from build123d import *

# Parameters (mm, degrees)
SKETCH_1_W               = 250
SKETCH_1_H               = 250
EXTRUDE_1_DEPTH          = 2
SKETCH_2_W               = 250
SKETCH_2_H               = 125
CUT_EXTRUDE_1_DEPTH      = 2
SKETCH_6_W               = 10
SKETCH_6_H               = 10
EXTRUDE_3_DEPTH          = 10
CUT_EXTRUDE_2_DEPTH      = 125
CUT_EXTRUDE_3_DEPTH      = 178.059312096
CUT_EXTRUDE_3_DEPTH_BACK = 178.059312096


with BuildPart() as part:
    # 草图1 → 凸台-拉伸1 (new body)
    with BuildSketch(Plane(origin=(0, 0, 0), x_dir=(1, 0, 0), z_dir=(0, 1, 0))):
        Rectangle(SKETCH_1_W, SKETCH_1_H)
    extrude(amount=EXTRUDE_1_DEPTH)

    # 草图2 → 切除-拉伸1 (cut)
    with BuildSketch(Plane(origin=(0, 2, 0), x_dir=(1, 0, 0), z_dir=(0, 1, 0))):
        with Locations((0, -62.5)):
            Rectangle(SKETCH_2_W, SKETCH_2_H)
    extrude(amount=-CUT_EXTRUDE_1_DEPTH, mode=Mode.SUBTRACT)

    # 草图6 → 凸台-拉伸3 (add)
    with BuildSketch(Plane.XZ):
        with Locations((-105.253353702, -19.703268914)):
            Rectangle(SKETCH_6_W, SKETCH_6_H)
        with Locations((-105.253353702, -104.703268914)):
            Rectangle(SKETCH_6_W, SKETCH_6_H)
        with Locations((104.746646298, -19.703268914)):
            Rectangle(SKETCH_6_W, SKETCH_6_H)
        with Locations((104.746646298, -104.703268914)):
            Rectangle(SKETCH_6_W, SKETCH_6_H)
    extrude(amount=EXTRUDE_3_DEPTH)

    # 草图9 → 切除-拉伸2 (cut)
    with BuildSketch(Plane(origin=(0, 0, -125), x_dir=(-1, 0, 0), z_dir=(0, 0, -1))):
        Polygon((-125, 0), (-125, 2), (-121.535898385, 2), align=None)
        Polygon((125, 2), (121.535898385, 2), (125, 0), align=None)
    extrude(amount=-CUT_EXTRUDE_2_DEPTH, mode=Mode.SUBTRACT)

    # 草图11 → 切除-拉伸3 (cut, two sides: drawn at the far end of the back side and taken through both)
    with BuildSketch(Plane(origin=(0, 0, 0), x_dir=(0, 0, -1), z_dir=(1, 0, 0)).offset(-CUT_EXTRUDE_3_DEPTH_BACK)):
        Polygon((0, 2), (0, 0), (3.464101615, 2), align=None)
    extrude(amount=CUT_EXTRUDE_3_DEPTH + CUT_EXTRUDE_3_DEPTH_BACK, mode=Mode.SUBTRACT)


solid = part.part
Geometry check sheet. Reference: the model listing, model coordinates, mm. A direction names the side the tool comes from. Coordinates: 2 decimals unless noted, no trailing zeros. Loops run counter-clockwise (first coordinate to the right, second up) from the corner with the lowest first, then second, coordinate; pieces in that order, holes last. Notation, with made-up numbers: (39.5, -1.75) - (81.5, -1.75) arc R23 ccw to (81.5, 28.25) - close; hole circle Ø1 at (63.5, 65.25). An arc over 180 degrees is marked (long way). Use one line per item in the form item = value. Start each with the question number.
Item 1: Tool access check on faces 5 (the face through (-105, -5, -14.703)), 6 (the face through (105, -5, -109.703)), 7 (the face through (-110.253, -5, -105)), 8 (the face through (105, -5, -24.703)), 9 (the face through (109.747, -5, -20)). Record the directions out of +Z, -Z, +X, -X, +Y, -Y that give a thin tool (end or side, any length) a straight path to the whole face; none if there is none.
Item 2: Section check D-D, the plane z = -94.5. Enter the section's corners in (x, y).
Item 3: Section check C-C, the plane x = 96.5. Enter the section's corners in (y, z).
Item 4: Section check A-A, the plane y = -4. Enter the section's corners in (x, z).
Item 5: Thickness scan on probe 1 along X at (y, z) = (-5.5, -103.5); probe 2 along Z at (x, y) = (-101, -2.5); probe 3 along Y at (x, z) = (-67.5, -67.5). Record the ranges inside material, lowest first.
Item 6: Section check B-B, the plane z = -22. Enter the section's corners in (x, y), and give its area (3 significant figures).
Item 7: Mould release check, pull along X, two halves, no side actions. Record for faces 1 (the face through (-110.253, -5, -20)), 2 (the face through (-100.253, -5, -105)), 3 (the face through (99.747, -5, -20)), 4 (the face through (105, -10, -20)): +X half, -X half, draft (parallel to the pull), parting line (faces both ways), or undercut.
Item 8: Gauge pin test, flat ends, axial feed: pin 1 (1 mm diameter, centred on y = -3, z = -102.5, fed in from +X); pin 2 (1.5 mm diameter, centred on y = 0, z = -31, fed in from -X); pin 3 (12 mm diameter, centred on x = 35.5, z = -53.5, fed in from -Y). Record the tip position at first contact, or that the pin passes through.
Computed:
q1.face_5 = +Z, +X, -X, -Y
q1.face_6 = -Z, +X, -X, -Y
q1.face_7 = +Z, -Z, -X, -Y
q1.face_8 = +X, -X, -Y
q1.face_9 = +Z, -Z, +X, -Y
q2.outline = (-125, 0) - (125, 0) - (121.54, 2) - (-121.54, 2) - close
q3.outline = (0, -125) - (2, -125) - (2, -3.46) - (0, 0) - close
q4.outline = (-110.25, -109.7) - (-100.25, -109.7) - (-100.25, -99.7) - (-110.25, -99.7) - close; (-110.25, -24.7) - (-100.25, -24.7) - (-100.25, -14.7) - (-110.25, -14.7) - close; (99.75, -109.7) - (109.75, -109.7) - (109.75, -99.7) - (99.75, -99.7) - close; (99.75, -24.7) - (109.75, -24.7) - (109.75, -14.7) - (99.75, -14.7) - close
q5.probe_1 = -110.25 to -100.25, 99.75 to 109.75
q5.probe_2 = -109.7 to -99.7, -24.7 to -14.7
q5.probe_3 = 0 to 2
q6.outline = (-125, 0) - (-110.25, 0) - (-110.25, -10) - (-100.25, -10) - (-100.25, 0) - (99.75, 0) - (99.75, -10) - (109.75, -10) - (109.75, 0) - (125, 0) - (121.54, 2) - (-121.54, 2) - close
q6.area = 693 mm2
q7.face_1 = -X half
q7.face_2 = undercut
q7.face_3 = undercut
q7.face_4 = draft
q8.pin_1 = 109.75
q8.pin_2 = -125
q8.pin_3 = 0
